from build123d import *

# Parameters (mm, degrees)
SKETCH1_R           = 30
SKETCH1_R_2         = 15
BOSS_EXTRUDE1_DEPTH = 40
SKETCH2_R           = 9.5
CUT_EXTRUDE1_DEPTH  = 2.5
SKETCH3_R           = 8.25
CUT_EXTRUDE2_DEPTH  = 15
CIRPATTERN1_COUNT   = 4
SKETCH4_R           = 2.5
CUT_EXTRUDE3_DEPTH  = 47.904157769


with BuildPart() as part:
    # Sketch1 → Boss-Extrude1 (new body)
    with BuildSketch(Plane(origin=(0, 0, 0), x_dir=(0, 0, -1), z_dir=(1, 0, 0))):
        Circle(SKETCH1_R)
        Circle(SKETCH1_R_2, mode=Mode.SUBTRACT)
    extrude(amount=BOSS_EXTRUDE1_DEPTH)

    # Sketch2 → Cut-Extrude1 (cut, symmetric)
    with BuildSketch(Plane.XY.offset(22)):
        with Locations((20, 0)):
            Circle(SKETCH2_R)
    cut_extrude1 = extrude(amount=CUT_EXTRUDE1_DEPTH, both=True, mode=Mode.SUBTRACT)

    # Sketch3 → Cut-Extrude2 (cut, symmetric)
    with BuildSketch(Plane.XY.offset(22)):
        with Locations((20, 0)):
            Circle(SKETCH3_R)
    cut_extrude2 = extrude(amount=CUT_EXTRUDE2_DEPTH, both=True, mode=Mode.SUBTRACT)

    # CirPattern1: Cut-Extrude1, Cut-Extrude2 ×4 about axis
    cirpattern1_axis = Axis((0, 0, 0), (1, 0, 0))
    add([cut_extrude1.rotate(cirpattern1_axis, i * 360 / CIRPATTERN1_COUNT) for i in range(1, CIRPATTERN1_COUNT)], mode=Mode.SUBTRACT)
    add([cut_extrude2.rotate(cirpattern1_axis, i * 360 / CIRPATTERN1_COUNT) for i in range(1, CIRPATTERN1_COUNT)], mode=Mode.SUBTRACT)


with BuildPart() as body_2:
    # Split2: the piece on the far side of the plane
    add(part.part)
    split(bisect_by=Plane(origin=(20, 0, 0), x_dir=(0, 0, 1), z_dir=(1, 0, 0)), keep=Keep.BOTTOM)


with BuildPart() as part_1:
    add(part.part)

    # Split2
    split(bisect_by=Plane(origin=(20, 0, 0), x_dir=(0, 0, 1), z_dir=(1, 0, 0)), keep=Keep.TOP)

    # Sketch4 → Cut-Extrude3 (cut, through all)
    with BuildSketch(Plane(origin=(40, 0, 0), x_dir=(0, 0, -1), z_dir=(1, 0, 0))):
        with Locations((-17.67766953, 17.67766953)):
            Circle(SKETCH4_R)
        with Locations((16.970562748, 16.970562748)):
            Circle(SKETCH4_R)
        with Locations((16.263455967, -17.67766953)):
            Circle(SKETCH4_R)
        with Locations((-18.384776311, -16.970562748)):
            Circle(SKETCH4_R)
    extrude(amount=-CUT_EXTRUDE3_DEPTH, mode=Mode.SUBTRACT)


solid = part_1.part
Verification items for the finished model (mm, model axes). A direction names the side the tool comes from. Give positions to 0.01 mm unless a question says otherwise; leave off trailing zeros. Order: outer loops, then holes, each group sorted by start corner. A loop starts at its lowest first (then second) coordinate and runs counter-clockwise, first axis right, second up. Notation, with made-up numbers: M 87.5,-29.75 L 130.5,-29.75 A8 ccw 130.5,-23.75 Z; hole C -37,67 d7. An arc over 180 degrees is marked long. Answer as a JSON object with one key per item and string values. Group by question number.
1) Access from +Z, -Z, +X, -X, +Y, -Y to the whole of each face (thin tool, end or side, straight path). Record for faces 4 (the face through (28.25, -0.18, 16.84)), 5 (the face through (29, -24.5, -1)).
2) Cross-section at A-A (y = 0). Enter the section's corners in (x, z), then the cut area to 3 significant figures.
3) Cross-section at C-C (y = -18.5). Enter the section's corners in (x, z).
4) Scan lines: line 1 along Y through (x, z) = (27, 17); line 2 along Y through (x, z) = (28.25, -10.5); line 3 along Z through (x, y) = (27.5, -13.5). Record each from-to range of solid material in increasing order. Write a range as [from, to].
5) Cross-section at D-D (x = 27.5). Give the number of separate pieces and of enclosed holes in the cut face, then the cut area to 3 significant figures.
6) Depth check by flat-ended pin: pin 1 Ø10.5 at (x, z) = (26.5, -4) entering from -Y; pin 2 Ø5 at (x, y) = (29, -4) entering from -Z; pin 3 Ø5 at (x, y) = (27, 4.5) entering from -Z; pin 4 Ø6 at (x, z) = (35, 9.5) entering from +Y. Enter the tip coordinate at first touch or a pass-through.
7) Mould release check, pull along Y, two halves, no side actions. Record for faces 1 (the face through (29.86, -11.49, -27.712)), 2 (the face through (30.14, 15.449, -14.987)), 3 (the face through (20, -16, -19)): released by +Y, released by -Y, zero draft, split by the parting line, or undercut.
Result sheet:
{
 "1": {"face 4": "+Z, -Z, -X", "face 5": "-X"},
 "2": {"outline": "M 28.25,-30 L 40,-30 L 40,-15 L 28.25,-15 L 28.25,-19.5 L 29.5,-19.5 L 29.5,-24.5 L 28.25,-24.5 Z; M 28.25,15 L 40,15 L 40,30 L 28.25,30 L 28.25,24.5 L 29.5,24.5 L 29.5,19.5 L 28.25,19.5 Z", "area": "340 mm2"},
 "3": {"outline": "M 20,-23.62 L 40,-23.62 L 40,-18.62 L 20,-18.62 Z; M 20,-13.9 L 40,-13.9 L 40,16.41 L 20,16.41 L 20,8.25 A8.25 cw 20,-8.25 Z; M 20,20.36 L 40,20.36 L 40,23.62 L 20,23.62 Z"},
 "4": {"line 1": "y = [-24.72, -19.05], [-14.89, -4.37], [4.37, 15.27], [20.08, 24.72]", "line 2": "y = [-28.1, -10.71], [10.71, 28.1]", "line 3": "z = [-26.79, -6.54], [6.54, 26.79]"},
 "5": {"separate pieces": "4", "enclosed holes": "4", "area": "1,530 mm2"},
 "6": {"pin 1": "stops at y = -30", "pin 2": "stops at z = -29.96", "pin 3": "stops at z = -29.92", "pin 4": "stops at y = 29.29"},
 "7": {"face 1": "split by the parting line", "face 2": "undercut", "face 3": "zero draft"}
}
